```python
from build123d import *

# Parameters (mm, degrees)
CROQUIS1_W              = 35
CROQUIS1_H              = 35
SALIENTE_EXTRUIR2_DEPTH = 75.5
CROQUIS2_W              = 26.5
CROQUIS2_H              = 26.5
CORTAR_EXTRUIR1_DEPTH   = 80
CROQUIS4_R              = 1.25
CORTAR_EXTRUIR2_DEPTH   = 10
CROQUIS6_W              = 26.5
CROQUIS6_H              = 26.5
SALIENTE_EXTRUIR3_DEPTH = 30
CORTAR_EXTRUIR3_DEPTH   = 27
CROQUIS8_W              = 26.5
CROQUIS8_H              = 26.5
CORTAR_EXTRUIR4_DEPTH   = 23
CORTAR_EXTRUIR5_START   = -10
CROQUIS9_R              = 1.25
CORTAR_EXTRUIR5_DEPTH   = 10


with BuildPart() as part:
    # Croquis1 → Saliente-Extruir2 (new body)
    with BuildSketch(Plane.XY):
        Rectangle(CROQUIS1_W, CROQUIS1_H)
    extrude(amount=SALIENTE_EXTRUIR2_DEPTH)

    # Croquis2 → Cortar-Extruir1 (cut)
    with BuildSketch(Plane.XY.offset(75.5)):
        Rectangle(CROQUIS2_W, CROQUIS2_H)
    extrude(amount=-CORTAR_EXTRUIR1_DEPTH, mode=Mode.SUBTRACT)

    # Croquis4 → Cortar-Extruir2 (cut)
    with BuildSketch(Plane.XY.offset(75.5)):
        with Locations((-15.375, 15.38)):
            Circle(CROQUIS4_R)
        with Locations((15.38, 15.38)):
            Circle(CROQUIS4_R)
        with Locations((15.38, -15.38)):
            Circle(CROQUIS4_R)
        with Locations((-15.375, -15.38)):
            Circle(CROQUIS4_R)
    extrude(amount=-CORTAR_EXTRUIR2_DEPTH, mode=Mode.SUBTRACT)

    # Croquis6 → Saliente-Extruir3 (add)
    with BuildSketch(Plane.XY.offset(7)):
        Rectangle(CROQUIS6_W, CROQUIS6_H)
    extrude(amount=SALIENTE_EXTRUIR3_DEPTH)

    # Croquis7 → Cortar-Extruir3 (cut)
    with BuildSketch(Plane.XY.offset(37)):
        with BuildLine():
            Line((13.25, -5), (13.25, 5))
            Line((13.25, 5), (8.385525636, 9.270003226))
            ThreePointArc((8.385525636, 9.270003226), (0, 12.428301163), (-8.385525636, 9.270003226))
            Line((-8.385525636, 9.270003226), (-13.25, 5))
            Line((-13.25, 5), (-13.25, -5))
            Line((-13.25, -5), (-8.385525636, -9.270003226))
            ThreePointArc((-8.385525636, -9.270003226), (0, -12.428301163), (8.385525636, -9.270003226))
            Line((8.385525636, -9.270003226), (13.25, -5))
        make_face()
    extrude(amount=-CORTAR_EXTRUIR3_DEPTH, mode=Mode.SUBTRACT)

    # Croquis8 → Cortar-Extruir4 (cut)
    with BuildSketch(Plane(origin=(0, 0, 7), x_dir=(-1, 0, 0), z_dir=(0, 0, -1))):
        Rectangle(CROQUIS8_W, CROQUIS8_H)
    extrude(amount=-CORTAR_EXTRUIR4_DEPTH, mode=Mode.SUBTRACT)

    # Croquis9 → Cortar-Extruir5 (cut)
    with BuildSketch(Plane(origin=(0, 0, 0), x_dir=(-1, 0, 0), z_dir=(0, 0, -1)).offset(CORTAR_EXTRUIR5_START)):
        with Locations(Location((-15.38, 15.38, 0), (0, 0, 180))):
            Circle(CROQUIS9_R)
        with Locations((15.38, 15.38)):
            Circle(CROQUIS9_R)
        with Locations((15.38, -15.38)):
            Circle(CROQUIS9_R)
        with Locations(Location((-15.38, -15.38, 0), (0, 0, 180))):
            Circle(CROQUIS9_R)
    extrude(amount=CORTAR_EXTRUIR5_DEPTH, mode=Mode.SUBTRACT)


solid = part.part
```
Here's how the part is built. I have some questions about the finished solid (model axes, mm). A direction names the side the tool comes from. Give positions to 0.01 mm unless a question says otherwise; leave off trailing zeros. Loops run counter-clockwise (first coordinate to the right, second up) from the corner with the lowest first, then second, coordinate; pieces in that order, holes last. Notation, with made-up numbers: M -7,82 L 40,82 A18 ccw 40,110 Z; hole C 38,26.5 d7. An arc over 180 degrees is marked long. Put each result on its own line as item: value. Start each with the question number.
(1) If we mould it in two halves opening along X, with no side actions, what happens to faces 1 (the flat face through (-15, -15, 65.5)), 2 (the flat face through (17.5, 0, 37)), 3 (the flat face through (-1, 14, 75.5))? For each: +X half, -X half, draft (parallel to the pull), parting line (faces both ways), or undercut.
(2) I want a section at D-D on x = -3.5. Please give me the cut outline in (y, z).
(3) For faces 4 (the flat face through (0, 13, 37)), 5 (the flat face through (-13.25, 0, 38)), 6 (the cylindrical face through (-16.57, 15.76, 5.07)), 7 (the flat face through (10.852, 7.105, 33.549)), which set-ups out of +Z, -Z, +X, -X, +Y, -Y let a thin tool reach every point of the face, with its end or its side?
(4) I need wall thicknesses on line 1 along Y through (x, z) = (-15.38, 6.25); line 2 along X through (y, z) = (-11.5, 15.5). Which ranges of each line are inside material? Lowest first, please. Write a range as [from, to].
(5) Will these pins go through, and if not, where does the flat tip stop? pin 1 Ø0.8 at (x, y) = (15, 15.5) entering from -Z; pin 2 Ø4 at (x, y) = (-15.375, 15.38) entering from +Z; pin 3 Ø2 at (x, y) = (15.38, 15.38) entering from +Z; pin 4 Ø1.5 at (x, y) = (-12, -8.5) entering from +Z.
(6) I want a section at B-B on y = 15.38. Please give me the cut outline in (x, z) (3 decimals), then the cut area to 3 significant figures.
(7) I want a section at C-C on z = 66.5. Please give me the cut outline in (x, y) (3 decimals).
(8) I want a section at A-A on z = 11. Please give me the cut outline in (x, y).
Answer block:
1. face 1: undercut
1. face 2: +X half
1. face 3: draft
2. outline: M -17.5,0 L -13.25,0 L -13.25,30 L -11.94,30 L -11.94,37 L -13.25,37 L -13.25,75.5 L -17.5,75.5 Z; M 11.94,30 L 13.25,30 L 13.25,0 L 17.5,0 L 17.5,75.5 L 13.25,75.5 L 13.25,37 L 11.94,37 Z
3. face 4: +Z
3. face 5: none
3. face 6: -Z
3. face 7: +Z, -Z
4. line 1: [-17.5, -16.63], [-14.13, 14.13], [16.63, 17.5]
4. line 2: [-17.5, -13.25], [13.25, 17.5]
5. pin 1: z = 10
5. pin 2: z = 75.5
5. pin 3: z = 65.5
5. pin 4: z = 37
6. outline: M -17.5,0 L -16.63,0 L -16.63,10 L -14.13,10 L -14.13,0 L 14.13,0 L 14.13,10 L 16.63,10 L 16.63,0 L 17.5,0 L 17.5,75.5 L 16.63,75.5 L 16.63,65.5 L 14.13,65.5 L 14.13,75.5 L -14.125,75.5 L -14.125,65.5 L -16.625,65.5 L -16.625,75.5 L -17.5,75.5 Z
6. area: 2,540 mm^2
7. outline: M -17.5,-17.5 L 17.5,-17.5 L 17.5,17.5 L -17.5,17.5 Z; hole C -15.375,-15.38 d2.5; hole C -15.375,15.38 d2.5; hole M -13.25,-13.25 L 13.25,-13.25 L 13.25,13.25 L -13.25,13.25 Z; hole C 15.38,-15.38 d2.5; hole C 15.38,15.38 d2.5
8. outline: M -17.5,-17.5 L 17.5,-17.5 L 17.5,17.5 L -17.5,17.5 Z; hole M -13.25,-13.25 L 13.25,-13.25 L 13.25,13.25 L -13.25,13.25 Z
